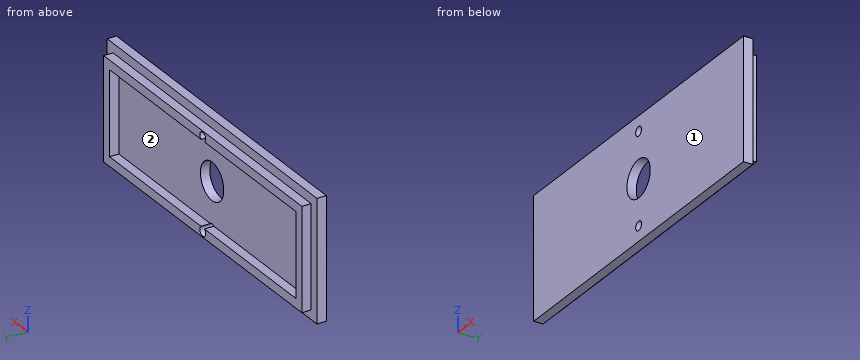
Autodesk Inventor part; units mm, degrees
ref_plane "YZ Plane" through (0, 0, 0) normal (1, 0, 0) x (0, 1, 0)
ref_plane "XZ Plane" through (0, 0, 0) normal (0, 1, 0) x (-1, 0, 0)
ref_plane "XY Plane" through (0, 0, 0) normal (0, 0, 1) x (1, 0, 0)
sketch "Sketch1" plane through (0, 0, 0) normal (0, 1, 0) x (-1, 0, 0)
  line L0 (74.4424, -50.7093) -> (-39.8576, -50.7093)
  line L1 (-39.8576, -50.7093) -> (-39.8576, -9.4343)
  line L2 (-39.8576, -9.4343) -> (74.4424, -9.4343)
  line L3 (74.4424, -9.4343) -> (74.4424, -50.7093)
  point P0 (0, 0)
  dimension "d0" = 41.275
  dimension "d1" = 114.3
extrude "Extrusion1" add sketch "Sketch1" along normal blind 3.175
sketch "Sketch2" plane through (0, 3.175, 0) normal (0, 1, 0) x (1, 0, 0)
  line L0 (-74.4424, 50.7093) -> (-74.4424, 9.4343)
  line L1 (-74.4424, 50.7093) -> (-71.2674, 50.7093)
  line L2 (39.8576, 50.7093) -> (-74.4424, 50.7093)
  line L3 (-71.2674, 50.7093) -> (-71.2674, 47.5343)
  line L4 (-71.2674, 47.5343) -> (-68.0924, 47.5343)
  line L5 (-68.0924, 47.5343) -> (-68.0924, 12.6093)
  line L6 (-68.0924, 12.6093) -> (-71.2674, 12.6093)
  line L7 (-71.2674, 12.6093) -> (-71.2674, 47.5343)
  point P0 (0, 0)
  dimension "d4" = 3.175
  dimension "d5" = 3.175
  dimension "d6" = 3.175
  dimension "d7" = 34.925
extrude "Extrusion2" add sketch "Sketch2" along normal blind 3.175
sketch "Sketch3" plane through (0, 3.175, 0) normal (0, 1, 0) x (1, 0, 0)
  line L0 (39.8576, 9.4343) -> (39.8576, 50.7093)
  line L1 (39.8576, 50.7093) -> (36.6826, 50.7093)
  line L2 (39.8576, 50.7093) -> (-74.4424, 50.7093)
  line L3 (36.6826, 50.7093) -> (36.6826, 47.5343)
  line L4 (36.6826, 47.5343) -> (33.5076, 47.5343)
  line L5 (33.5076, 47.5343) -> (33.5076, 12.6093)
  line L6 (33.5076, 12.6093) -> (36.6826, 12.6093)
  line L7 (36.6826, 12.6093) -> (36.6826, 47.5343)
  point P0 (0, 0)
  dimension "d10" = 3.175
  dimension "d11" = 3.175
  dimension "d12" = 3.175
  dimension "d13" = 34.925
extrude "Extrusion3" add sketch "Sketch3" along normal blind 3.175
sketch "Sketch4" plane through (0, 3.175, 0) normal (0, 1, 0) x (1, 0, 0)
  line L0 (-68.0924, 47.5343) -> (-68.0924, 12.6093)
  line L1 (-68.0924, 47.5343) -> (33.5076, 47.5343)
  line L2 (33.5076, 47.5343) -> (33.5076, 44.3593)
  line L3 (33.5076, 44.3593) -> (-68.0924, 44.3593)
  line L4 (-68.0924, 44.3593) -> (-68.0924, 47.5343)
  point P0 (0, 0)
  dimension "d16" = 3.175
  dimension "d17" = 101.6
extrude "Extrusion4" add sketch "Sketch4" along normal blind 3.175
sketch "Sketch5" plane through (0, 3.175, 0) normal (0, 1, 0) x (1, 0, 0)
  line L0 (-71.2674, 12.6093) -> (-68.0924, 12.6093)
  line L1 (-68.0924, 12.6093) -> (33.5076, 12.6093)
  line L2 (33.5076, 12.6093) -> (33.5076, 15.7843)
  line L3 (33.5076, 15.7843) -> (-68.0924, 15.7843)
  line L4 (-68.0924, 15.7843) -> (-68.0924, 12.6093)
  point P0 (0, 0)
  dimension "d20" = 3.175
  dimension "d21" = 101.6
extrude "Extrusion5" add sketch "Sketch5" along normal blind 3.175
sketch "Sketch10" plane through (0, 0, 0) normal (0, -1, 0) x (1, 0, 0)
  line L0 (39.8576, -9.4343) -> (39.8576, -30.0718)
  line L1 (39.8576, -9.4343) -> (39.8576, -50.7093)
  line L2 (39.8576, -30.0718) -> (-17.2924, -30.0718)
  point P0 (0, 0)
  dimension "d38" = 20.6375
  dimension "d39" = 57.15
hole "Hole2" at (-17.2924, 0, -30.0718) direction (0, 1, 0) diameter 12.7 end through all
sketch "Sketch13" plane through (0, 0, 0) normal (0, -1, 0) x (1, 0, 0)
  line L0 (39.8576, -9.4343) -> (39.8576, -50.7093)
  line L1 (39.8576, -9.4343) -> (39.8576, -14.5143)
  line L2 (39.8576, -14.5143) -> (-17.2924, -14.5143)
  point P0 (0, 0)
  dimension "d51" = 5.08
  dimension "d52" = 57.15
hole "Hole3" at (-17.2924, 0, -14.5143) direction (0, 1, 0) diameter 3.175 end through all
sketch "Sketch14" plane through (0, 0, 0) normal (0, -1, 0) x (1, 0, 0)
  line L0 (39.8576, -9.4343) -> (39.8576, -50.7093)
  line L1 (39.8576, -50.7093) -> (39.8576, -45.6293)
  line L2 (39.8576, -45.6293) -> (-17.2924, -45.6293)
  point P0 (0, 0)
  dimension "d60" = 5.08
  dimension "d61" = 57.15
hole "Hole4" at (-17.2924, 0, -45.6293) direction (0, 1, 0) diameter 3.175 end through all
properties part number "five_cell_top_case"
Work out the finished part from the listing and answer in its coordinate system (mm). Face numbers are marked on the shaded views. Give positions to 0.01 mm unless a question says otherwise; leave off trailing zeros. Order: outer loops, then holes, each group sorted by start corner. A loop starts at its lowest first (then second) coordinate and runs counter-clockwise, first axis right, second up.
1. Each of these flat-tipped pins is pushed along its axis until it touches: P1, Ø1.6, axis at x = 3.5, y = 5, coming from the +Z side; P2, Ø8.5, axis at x = -7.5, z = -23.5, coming from the +Y side (3 decimals); P3, Ø1, axis at x = -9.5, y = 4, coming from the -Z side; P4, Ø1.9, axis at x = -17.29, z = -45.63, coming from the -Y side. Where does it stop, or does it pass through?
Result sheet:
P1: stops at z = -12.61
P2: stops at y = 3.175
P3: stops at z = -47.53
P4: passes through
2. Section D-D, the plane z = -20.5 is taken. Determine the outline of the cut face in (x, y) (3 decimals).
Result sheet:
outline: (-74.442, 0) - (39.858, 0) - (39.858, 3.175) - (36.683, 3.175) - (36.683, 6.35) - (33.508, 6.35) - (33.508, 3.175) - (-68.092, 3.175) - (-68.092, 6.35) - (-71.267, 6.35) - (-71.267, 3.175) - (-74.442, 3.175) - close
3. Section A-A, the plane y = 4.5 is taken. Determine the outline of the cut face in (x, z) (1 decimal), and give its area (3 significant figures).
Result sheet:
outline: (-71.3, -47.5) - (36.7, -47.5) - (36.7, -12.6) - (-71.3, -12.6) - close; hole (-68.1, -44.4) - (-18.2, -44.4) arc R1.6 ccw (long way) to (-16.3, -44.4) - (33.5, -44.4) - (33.5, -15.8) - (-16.3, -15.8) arc R1.6 ccw (long way) to (-18.2, -15.8) - (-68.1, -15.8) - close
area: 852 mm2
4. Section B-B, the plane z = -30 is taken. Determine the outline of the cut face in (x, y) (3 decimals).
Result sheet:
outline: (-74.442, 0) - (-23.642, 0) - (-23.642, 3.175) - (-68.092, 3.175) - (-68.092, 6.35) - (-71.267, 6.35) - (-71.267, 3.175) - (-74.442, 3.175) - close; (-10.943, 0) - (39.858, 0) - (39.858, 3.175) - (36.683, 3.175) - (36.683, 6.35) - (33.508, 6.35) - (33.508, 3.175) - (-10.943, 3.175) - close
5. The mould has two halves that part along Z. Classify the marked faces 1 and 2: released by +Z, released by -Z, zero draft, split by the parting line, or undercut.
Result sheet:
face 1: zero draft
face 2: undercut
6. Section C-C, the plane x = 13 is taken. Determine the outline of the cut face in (y, z) (3 decimals), and give its area (3 significant figures).
Result sheet:
outline: (0, -50.709) - (3.175, -50.709) - (3.175, -47.534) - (6.35, -47.534) - (6.35, -44.359) - (3.175, -44.359) - (3.175, -15.784) - (6.35, -15.784) - (6.35, -12.609) - (3.175, -12.609) - (3.175, -9.434) - (0, -9.434) - close
area: 151 mm2
7. Straight lines are drawn through the part: L1, parallel to Z at x = 14, y = 4.75; L2, parallel to X at y = 5.25, z = -32; L3, parallel to Y at x = 8.5, z = -41 (3 decimals). For each, find the intervals that lie inside material, in ascending order.
Result sheet:
L1: z = -47.53 to -44.36, -15.78 to -12.61
L2: x = -71.27 to -68.09, 33.51 to 36.68
L3: y = 0 to 3.175
